Input: part model. Units: mm. Frame: model coordinates. Face numbers are marked on the shaded views. Give positions to 0.01 mm unless a question says otherwise; leave off trailing zeros. Order: outer loops, then holes, each group sorted by start corner. A loop starts at its lowest first (then second) coordinate and runs counter-clockwise, first axis right, second up. Notation, with made-up numbers: (45.25, -35.75) - (72.25, -35.75) arc R26 cw to (72.25, -2.75) - close; hole circle Ø9 at (35.25, 26.5). An arc over 180 degrees is marked (long way). Answer in a Markdown table with one row per item. Add a question column.
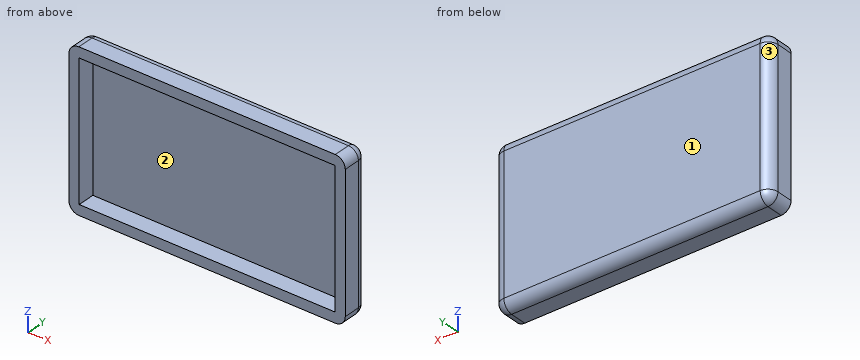
from build123d import *

# Parameters (mm, degrees)
SKETCH1_W           = 41.6
SKETCH1_H           = 23.6
BOSS_EXTRUDE1_DEPTH = 4
SKETCH2_W           = 38.5
SKETCH2_H           = 20.5
CUT_EXTRUDE1_DEPTH  = 2.6
FILLET1_R           = 1.5


with BuildPart() as part:
    # Sketch1 → Boss-Extrude1 (new body)
    with BuildSketch(Plane(origin=(0, 0, 0), x_dir=(1, 0, 0), z_dir=(0, 1, 0))):
        with Locations((20.8, 11.8)):
            Rectangle(SKETCH1_W, SKETCH1_H)
    extrude(amount=BOSS_EXTRUDE1_DEPTH)

    # Sketch2 → Cut-Extrude1 (cut)
    with BuildSketch(Plane.XZ):
        with Locations((20.8, -11.8)):
            Rectangle(SKETCH2_W, SKETCH2_H)
    extrude(amount=-CUT_EXTRUDE1_DEPTH, mode=Mode.SUBTRACT)

    # Fillet1
    fillet1_edges = [part.edges().sort_by_distance(p)[0] for p in [
        (41.6, 4, -11.8),
        (20.8, 4, -23.6),
        (0, 4, -11.8),
        (20.8, 4, 0),
        (0, 2, -23.6),
        (41.6, 2, -23.6),
        (41.6, 2, 0),
        (0, 2, 0),
    ]]
    fillet(fillet1_edges, radius=FILLET1_R)


solid = part.part
Q1. Section B-B, the plane z = -17.5. Return loops of the section in (x, y), then the cut area to 3 significant figures.
Q2. Section A-A, the plane y = 1.5. Return loops of the section in (x, z), then the cut area to 3 significant figures.
Q3. Contact query for a flat-ended pin moving along its axis: P1, Ø10, axis at x = 25.5, z = -15, coming from the -Y side. Output: stop coordinate, or through.
Q4. Section D-D, the plane y = 3.6. Return loops of the section in (x, z), then the cut area to 3 significant figures.
Q5. Line query: probe 1 along X at (y, z) = (1.35, -8.5); probe 2 along Z at (x, y) = (35, 1.45); probe 3 along Y at (x, z) = (34.5, -20.75). Output: solid intervals per line, ascending.
Q6. Pull-direction query (X, two-part tool) for the marked faces 1, 2 and 3; classes: +X half, -X half, draft (parallel to the pull), parting line (faces both ways), or undercut.
Q7. Section C-C, the plane x = 22. Return loops of the section in (y, z), then the cut area to 3 significant figures.
Computed:
| question | item | result |
|---|---|---|
| 1 | outline | (0, 0) - (1.55, 0) - (1.55, 2.6) - (40.05, 2.6) - (40.05, 0) - (41.6, 0) - (41.6, 2.5) arc R1.5 ccw to (40.1, 4) - (1.5, 4) arc R1.5 ccw to (0, 2.5) - close |
| 1 | area | 65.3 mm^2 |
| 2 | outline | (0, -22.1) arc R1.5 ccw to (1.5, -23.6) - (40.1, -23.6) arc R1.5 ccw to (41.6, -22.1) - (41.6, -1.5) arc R1.5 ccw to (40.1, 0) - (1.5, 0) arc R1.5 ccw to (0, -1.5) - close; hole (1.55, -22.05) - (40.05, -22.05) - (40.05, -1.55) - (1.55, -1.55) - close |
| 2 | area | 191 mm^2 |
| 3 | P1 | stops at y = 2.6 |
| 4 | outline | (0.48, -22.1) arc R1.02 ccw to (1.5, -23.12) - (40.1, -23.12) arc R1.02 ccw to (41.12, -22.1) - (41.12, -1.5) arc R1.02 ccw to (40.1, -0.48) - (1.5, -0.48) arc R1.02 ccw to (0.48, -1.5) - close |
| 4 | area | 919 mm^2 |
| 5 | probe 1 | x = 0 to 1.55, 40.05 to 41.6 |
| 5 | probe 2 | z = -23.6 to -22.05, -1.55 to 0 |
| 5 | probe 3 | y = 2.6 to 4 |
| 6 | face 1 | draft |
| 6 | face 2 | undercut |
| 6 | face 3 | -X half |
| 7 | outline | (0, -23.6) - (2.5, -23.6) arc R1.5 ccw to (4, -22.1) - (4, -1.5) arc R1.5 ccw to (2.5, 0) - (0, 0) - (0, -1.55) - (2.6, -1.55) - (2.6, -22.05) - (0, -22.05) - close |
| 7 | area | 40.1 mm^2 |
